Geometry: final body of the model. Coordinates: model frame, mm. Face numbers are marked on the shaded views. A direction names the side the tool comes from. Give positions to 0.01 mm unless a question says otherwise; leave off trailing zeros. Order: outer loops, then holes, each group sorted by start corner. A loop starts at its lowest first (then second) coordinate and runs counter-clockwise, first axis right, second up. Notation, with made-up numbers: (63, 88.25) - (83, 88.25) arc R26 ccw to (83, 116.25) - close; hole circle Ø2 at (42, 53.5). An arc over 180 degrees is marked (long way). Use one line per item in the form item = value.
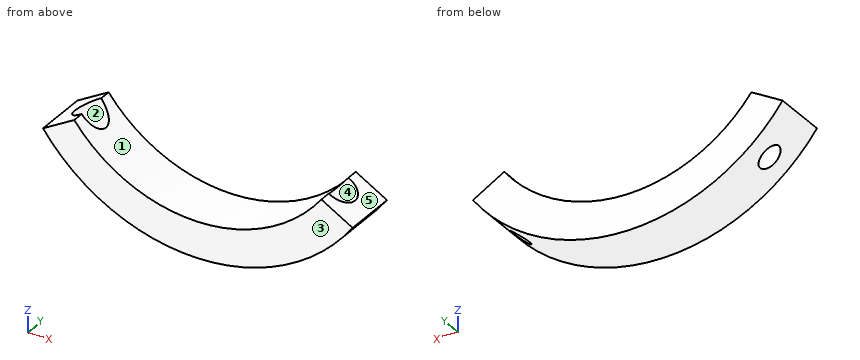
from build123d import *

# Parameters (mm, degrees)
F1_DEPTH = 17.5
F5_R     = 3
F6_DEPTH = 46.213747
F5_R_2   = 5
F7_DEPTH = 26


with BuildPart() as f1:
    # F0 (on Front) → F1 (new body)
    with BuildSketch(Plane.XZ):
        with BuildLine():
            ThreePointArc((39.686286, 4.873462), (0, -14.712747), (-39.686286, 4.873462))
            Line((-39.686286, 4.873462), (-49.714635, -0.916408))
            ThreePointArc((-49.714635, -0.916408), (0, -26.212747), (49.714635, -0.916408))
            Line((49.714635, -0.916408), (39.686286, 4.873462))
        make_face()
    extrude(amount=-F1_DEPTH)

    # F5 (on offset) → F6 (cut, through all)
    with BuildSketch(Plane.XY.offset(20)):
        with Locations((40, 8.75)):
            Circle(F5_R)
        with Locations((-40, 8.75)):
            Circle(F5_R)
    extrude(amount=-F6_DEPTH, mode=Mode.SUBTRACT)

    # F5 (on offset) → F7 (cut)
    with BuildSketch(Plane.XY.offset(20)):
        with Locations((40, 8.75)):
            Circle(F5_R_2)
        with Locations((40, 8.75)):
            Circle(F5_R, mode=Mode.SUBTRACT)
        with Locations((-40, 8.75)):
            Circle(F5_R_2)
        with Locations((-40, 8.75)):
            Circle(F5_R, mode=Mode.SUBTRACT)
    extrude(amount=-F7_DEPTH, mode=Mode.SUBTRACT)


with BuildPart() as f2_1:
    # F2: copy of F1
    add(f1.part)


solid = f1.part
(1) Contact query for flat-ended pins moving along their axis: pin 1 Ø3 at (y, z) = (5, -7) entering from +X; pin 2 Ø2 at (x, y) = (20.5, 13) entering from +Z; pin 3 Ø3 at (y, z) = (10.5, -14) entering from +X; pin 4 Ø5.5 at (x, y) = (40, 8.75) entering from -Z. Output: stop coordinate, or through.
Computed values:
pin_1 = 46.03
pin_2 = -9.85
pin_3 = 38.42
pin_4 = through
(2) Pull-direction query (Y, two-part tool) for the marked faces 3, 4 and 5; classes: released by +Y, released by -Y, zero draft, split by the parting line, or undercut.
Computed values:
face_3 = released by -Y
face_4 = undercut
face_5 = zero draft
(3) Cut plane D-D on y = 16.25. Output: boundary loops of the cut face in (x, z), plus the area to 3 significant figures.
Computed values:
outline = (-49.71, -0.92) arc R61.5 ccw to (49.71, -0.92) - (39.69, 4.87) arc R50 cw to (-39.69, 4.87) - close
area = 1,190 mm²
(4) Cut plane B-B on y = 8.75. Output: boundary loops of the cut face in (x, z).
Computed values:
outline = (-49.71, -0.92) arc R61.5 ccw to (-43, -8.68) - (-43, -6) - (-45, -6) - (-45, 1.81) - close; (-37, -13.84) arc R61.5 ccw to (37, -13.84) - (37, -6) - (35, -6) - (35, -0.42) arc R50 cw to (-35, -0.42) - (-35, -6) - (-37, -6) - close; (43, -8.68) arc R61.5 ccw to (49.71, -0.92) - (45, 1.81) - (45, -6) - (43, -6) - close
(5) Cut plane C-C on x = -42. Output: boundary loops of the cut face in (y, z), plus the area to 3 significant figures.
Computed values:
outline = (0, -9.64) - (6.51, -9.64) - (6.51, -6) - (4.17, -6) - (4.17, 3.54) - (0, 3.54) - close; (10.99, -9.64) - (17.5, -9.64) - (17.5, 3.54) - (13.33, 3.54) - (13.33, -6) - (10.99, -6) - close
area = 127 mm²
(6) Ray query, line 1 along Y through (x, z) = (-40, 0); line 2 along Y through (x, z) = (40, -10); line 3 along X through (y, z) = (8.75, -8.5). Return the intervals inside material, ascending.
Computed values:
line_1 = 0 to 3.75, 13.75 to 17.5
line_2 = 0 to 5.75, 11.75 to 17.5
line_3 = -43.18 to -43, -37 to -24.14, 24.14 to 37, 43 to 43.18
(7) Reachability of the marked faces 1 and 2 from +Z, -Z, +X, -X, +Y, -Y: full face, straight path, thin tool, end or side. Return the list, or none.
Computed values:
face_1 = +Z, +Y, -Y
face_2 = +Z
(8) Cut plane A-A on z = -7.5. Output: boundary loops of the cut face in (x, y), plus the area to 3 significant figures.
Computed values:
outline = (-44.18, 0) - (-25.87, 0) - (-25.87, 17.5) - (-44.18, 17.5) - close; (25.87, 0) - (44.18, 0) - (44.18, 17.5) - (25.87, 17.5) - close; hole circle Ø6 at (-40, 8.75); hole circle Ø6 at (40, 8.75)
area = 584 mm²
